```python
from build123d import *

# Parameters (mm, degrees)
F0_R     = 24.5
F1_DEPTH = 72
F2_T     = -2


# Not quite as in the source:
# - a fillet or chamfer that OpenCascade refuses, or shapes differently, is made with other operations: its cross-section is extruded or revolved along the edge and cut away or added


with BuildPart() as f1:
    # F0 (on Top) → F1 (new body)
    with BuildSketch(Plane.XY):
        Circle(F0_R)
    extrude(amount=F1_DEPTH)

    # F2
    f2_openings = [f1.faces().sort_by_distance(p)[0] for p in [
        (0, 0, 72),
    ]]
    offset(amount=F2_T, openings=f2_openings)

    # F3: chamfer of 5 on 1 edges, made by hand

    # F3_s1 → F3_t2 (revolve, cut)
    with BuildSketch(Plane.XZ):
        Polygon((27.5, 72), (22.5, 67), (22.5, 72), align=None)
    revolve(axis=Axis((0, 0, 72), (0, 0, 1)), mode=Mode.SUBTRACT)


solid = f1.part
```
CAD build for the part. Positions are in the model's coordinates, mm. Coordinates: 2 decimals unless noted, no trailing zeros. Write each loop counter-clockwise with the first axis right and the second up, starting at its lowest first coordinate (ties: lowest second). Pieces come first, ordered by that corner, then holes.
(1) Two-plate mould, pull along X, no slides. Class faces 1 (the face through (0, 0, 2)), 2 (the face through (13.17, 20.66, 34.02)), 3 (the face through (0, 0, 0)): +X half, -X half, draft (parallel to the pull), parting line (faces both ways), or undercut.
(2) Drill centre lines: probe 1 along Y at (x, z) = (0, 50); probe 2 along Z at (x, y) = (-7, 4). Where is each one in solid material? Low to high.
(3) Cut at A-A, the plane x = 0. List the corners of the cut face in (y, z).
(4) Cut at C-C, the plane z = 54.5. List the corners of the cut face in (x, y), and give its area (3 significant figures).
(5) Flat gauge pins, fed straight in: pin 1 (6 mm diameter, centred on x = 4, y = 1.5, fed in from +Z); pin 2 (10 mm diameter, centred on x = -1, z = 32, fed in from -Y); pin 3 (1.5 mm diameter, centred on x = 0.5, z = 52, fed in from +Y). Where does each tip first touch, or does it go through?
Geometry says:
1. face 1: undercut
1. face 2: parting line
1. face 3: draft
2. probe 1: y = -24.5 to -22.5, 22.5 to 24.5
2. probe 2: z = 0 to 2
3. outline: (-24.5, 0) - (24.5, 0) - (24.5, 69) - (22.5, 67) - (22.5, 2) - (-22.5, 2) - (-22.5, 67) - (-24.5, 69) - close
4. outline: circle Ø49 at (0, 0); hole circle Ø45 at (0, 0)
4. area: 295 mm2
5. pin 1: stops at z = 2
5. pin 2: stops at y = -24.5
5. pin 3: stops at y = 24.5
